CAD build for the part. Positions are in the model's coordinates, mm. A direction names the side the tool comes from. Coordinates: 2 decimals unless noted, no trailing zeros. Order: outer loops, then holes, each group sorted by start corner. A loop starts at its lowest first (then second) coordinate and runs counter-clockwise, first axis right, second up. Notation, with made-up numbers: (7.25, 76.5) - (29.25, 76.5) arc R36 ccw to (29.25, 114.5) - close; hole circle Ø11 at (38.5, 11.5). An arc over 180 degrees is marked (long way). Use one line per item in the form item = value.
```python
from build123d import *

# Parameters (mm, degrees)
SKETCH_1_R      = 3.4
EXTRUDE_1_DEPTH = 380


with BuildPart() as part:
    # 草图1 → 凸台-拉伸1 (new body)
    with BuildSketch(Plane.XY):
        Polygon((-4.1, 12.5), (-4.1, 15), (-8.25, 15), (-15, 15), (-15, 8.25), (-15, 4.1), (-12.5, 4.1), (-12.5, 8.25), (-9.664213562, 8.25), (-5.8, 4.385786438), (-5.8, -4.385786438), (-9.664213562, -8.25), (-12.5, -8.25), (-12.5, -4.1), (-15, -4.1), (-15, -8.25), (-15, -15), (-8.25, -15), (-4.1, -15), (-4.1, -12.5), (-8.25, -12.5), (-8.25, -9.664213562), (-4.385786438, -5.8), (4.385786438, -5.8), (8.25, -9.664213562), (8.25, -12.5), (4.1, -12.5), (4.1, -15), (8.25, -15), (15, -15), (21.75, -15), (25.9, -15), (25.9, -12.5), (21.75, -12.5), (21.75, -9.664213562), (25.614213562, -5.8), (34.385786438, -5.8), (38.25, -9.664213562), (38.25, -12.5), (34.1, -12.5), (34.1, -15), (38.25, -15), (45, -15), (45, -8.25), (45, -4.1), (42.5, -4.1), (42.5, -8.25), (39.664213562, -8.25), (35.8, -4.385786438), (35.8, 4.385786438), (39.664213562, 8.25), (42.5, 8.25), (42.5, 4.1), (45, 4.1), (45, 8.25), (45, 15), (38.25, 15), (34.1, 15), (34.1, 12.5), (38.25, 12.5), (38.25, 9.664213562), (34.385786438, 5.8), (25.614213562, 5.8), (21.75, 9.664213562), (21.75, 12.5), (25.9, 12.5), (25.9, 15), (21.75, 15), (15, 15), (8.25, 15), (4.1, 15), (4.1, 12.5), (8.25, 12.5), (8.25, 9.664213562), (4.385786438, 5.8), (-4.385786438, 5.8), (-8.25, 9.664213562), (-8.25, 12.5), align=None)
        Circle(SKETCH_1_R, mode=Mode.SUBTRACT)
        Polygon((9.664213562, -8.25), (5.8, -4.385786438), (5.8, 4.385786438), (9.664213562, 8.25), (9.664213562, 12.5), (20.335786438, 12.5), (20.335786438, 8.25), (24.2, 4.385786438), (24.2, -4.385786438), (20.335786438, -8.25), (20.335786438, -12.5), (9.664213562, -12.5), align=None, mode=Mode.SUBTRACT)
        with Locations((30, 0)):
            Circle(SKETCH_1_R, mode=Mode.SUBTRACT)
    extrude(amount=EXTRUDE_1_DEPTH)


solid = part.part
```
Item 1: Drop flat-ended pins along their axis: pin 1 (4 mm diameter, centred on x = -4, z = 215.5, fed in from -Y); pin 2 (2 mm diameter, centred on y = -0.5, z = 316.5, fed in from +X); pin 3 (2.5 mm diameter, centred on y = 2, z = 264, fed in from -X). Give the stop position or say it passes through.
Derived:
pin_1 = -15
pin_2 = 35.8
pin_3 = -5.8
Item 2: Cut at B-B, the plane x = 17. Write the cut outline in (y, z).
Derived:
outline = (-15, 0) - (-12.5, 0) - (-12.5, 380) - (-15, 380) - close; (12.5, 0) - (15, 0) - (15, 380) - (12.5, 380) - close
Item 3: Cut at A-A, the plane y = 0. Write the cut outline in (x, z).
Derived:
outline = (-5.8, 0) - (-3.4, 0) - (-3.4, 380) - (-5.8, 380) - close; (3.4, 0) - (5.8, 0) - (5.8, 380) - (3.4, 380) - close; (24.2, 0) - (26.6, 0) - (26.6, 380) - (24.2, 380) - close; (33.4, 0) - (35.8, 0) - (35.8, 380) - (33.4, 380) - close
Item 4: Cut at C-C, the plane x = 0. Write the cut outline in (y, z).
Derived:
outline = (-5.8, 0) - (-3.4, 0) - (-3.4, 380) - (-5.8, 380) - close; (3.4, 0) - (5.8, 0) - (5.8, 380) - (3.4, 380) - close
Item 5: Drill centre lines: line 1 (X direction, y = 11.5, z = 323.5); line 2 (X direction, y = 4.25, z = 174); line 3 (Y direction, x = 0, z = 86.5). Where is each one in solid material? Low to high. Write a range as [from, to].
Derived:
line_1 = [-15, -8.25], [8.25, 9.66], [20.34, 21.75], [38.25, 45]
line_2 = [-15, -12.5], [-5.8, 5.8], [24.2, 35.8], [42.5, 45]
line_3 = [-5.8, -3.4], [3.4, 5.8]
Item 6: 3-axis set-ups, long thin cutter, end or side, ignore diameter. For faces 4 (the face through (15, -12.5, 187)), 5 (the face through (15, -15, 187)): which of +Z, -Z, +X, -X, +Y, -Y reach the whole face in a straight line?
Derived:
face_4 = +Z, -Z
face_5 = +Z, -Z, +X, -X, -Y
Item 7: Cut at D-D, the plane z = 227. State how many separate pieces and enclosed holes the cut face has, plus the area to 3 significant figures.
Derived:
separate_pieces = 1
enclosed_holes = 3
area = 666 mm²
Item 8: Two-plate mould, pull along Y, no slides. Class faces 1 (the face through (8, 7, 0)), 2 (the face through (39, -15, 187)), 3 (the face through (15, 12.5, 187)): +Y half, -Y half, draft (parallel to the pull), parting line (faces both ways), or undercut.
Derived:
face_1 = draft
face_2 = -Y half
face_3 = undercut
